Part model, mm, in its own coordinate system. A direction names the side the tool comes from. Coordinates: 2 decimals unless noted, no trailing zeros. Loops run counter-clockwise (first coordinate to the right, second up) from the corner with the lowest first, then second, coordinate; pieces in that order, holes last. Notation, with made-up numbers: M 32.25,24.5 L 36.25,24.5 A23 cw 36.25,38.5 Z; hole C 23.5,-9 d2. An arc over 180 degrees is marked long. Answer as a JSON object with one key per item and string values. Group by question number.
1. 3-axis set-ups, long thin cutter, end or side, ignore diameter. For faces 1 (the face through (2, 5, 1)), 2 (the face through (6, 7, 48.2)), 3 (the face through (-0.92, 7.04, 54.51)): which of +Z, -Z, +X, -X, +Y, -Y reach the whole face in a straight line?
2. Saw through at A-A on z = 13. Write the cut outline in (x, y).
3. Drill centre lines: L1, parallel to Y at x = -2.25, z = 41; L2, parallel to X at y = -0.75, z = 39; L3, parallel to Y at x = 2.75, z = 4.5. Where is each one in solid material? Low to high.
4. Mould opens along Y. For faces 4 (the face through (-1.08, -4.88, 27.13)), 5 (the face through (6, 7, 6.8)), 6 (the face through (4.38, -8.43, 3.22)) say: released by +Y, released by -Y, zero draft, split by the parting line, or undercut.
5. Drop flat-ended pins along their axis: pin 1 Ø6 at (x, z) = (-7, 19.5) entering from +Y; pin 2 Ø1 at (x, y) = (-6, -2.5) entering from +Z; pin 3 Ø3 at (y, z) = (0.5, 47) entering from -X; pin 4 Ø8.5 at (x, y) = (0, 0) entering from -Z. Give the stop position or say it passes through.
from build123d import *

# Parameters (mm, degrees)
SKETCH1_R           = 9.5
SKETCH1_R_2         = 5
BOSS_EXTRUDE1_DEPTH = 55
SKETCH2_R           = 7.1
CUT_EXTRUDE1_DEPTH  = 1
SKETCH3_R           = 7.1
CUT_EXTRUDE2_DEPTH  = 1
SKETCH4_W           = 0.5
SKETCH4_H           = 1.3
FILLET1_R           = 1


with BuildPart() as part:
    # Sketch1 → Boss-Extrude1 (new body)
    with BuildSketch(Plane.XY):
        Circle(SKETCH1_R)
        Circle(SKETCH1_R_2, mode=Mode.SUBTRACT)
    extrude(amount=BOSS_EXTRUDE1_DEPTH)

    # Sketch2 → Cut-Extrude1 (cut)
    with BuildSketch(Plane.XY.offset(55)):
        Circle(SKETCH2_R)
    extrude(amount=-CUT_EXTRUDE1_DEPTH, mode=Mode.SUBTRACT)

    # Sketch3 → Cut-Extrude2 (cut)
    with BuildSketch(Plane(origin=(0, 0, 0), x_dir=(-1, 0, 0), z_dir=(0, 0, -1))):
        Circle(SKETCH3_R)
    extrude(amount=-CUT_EXTRUDE2_DEPTH, mode=Mode.SUBTRACT)

    # Sketch4 → Cut-Revolve1 (revolve, cut)
    with BuildSketch(Plane(origin=(0, 0, 0), x_dir=(1, 0, 0), z_dir=(0, 1, 0))):
        with Locations((-9.25, -48.85)):
            Rectangle(SKETCH4_W, SKETCH4_H)
        with Locations((-9.25, -6.15)):
            Rectangle(SKETCH4_W, SKETCH4_H)
    revolve(axis=Axis((0, 0, 0), (0, 0, 1)), mode=Mode.SUBTRACT)

    # Fillet1
    fillet1_edges = [part.edges().sort_by_distance(p)[0] for p in [
        (-9.5, 0, 0),
        (-9.5, 0, 55),
    ]]
    fillet(fillet1_edges, radius=FILLET1_R)


solid = part.part
Outcome:
{
 "1": {"face 1": "-Z", "face 2": "none", "face 3": "+Z"},
 "2": {"outline": "C 0,0 d19; hole C 0,0 d10"},
 "3": {"L1": "y = -9.23 to -4.47, 4.47 to 9.23", "L2": "x = -9.47 to -4.94, 4.94 to 9.47", "L3": "y = -9.09 to -4.18, 4.18 to 9.09"},
 "4": {"face 4": "undercut", "face 5": "zero draft", "face 6": "split by the parting line"},
 "5": {"pin 1": "stops at y = 8.62", "pin 2": "stops at z = 54", "pin 3": "stops at x = -9.5", "pin 4": "passes through"}
}
